Print and shaded views of the part. All mm, measured from the part's lowest x, y and z. A direction names the side the tool comes from. Give positions to 0.01 mm unless a question says otherwise; leave off trailing zeros. Loops run counter-clockwise (first coordinate to the right, second up) from the corner with the lowest first, then second, coordinate; pieces in that order, holes last. Notation, with made-up numbers: (-4.5, 4) -> (43.5, 4) arc R8 ccw to (43.5, 17) -> close; hole circle Ø5 at (7.5, 14). An arc over 180 degrees is marked (long way). Answer as a JSON object with one key per item and string values. Group by question number.
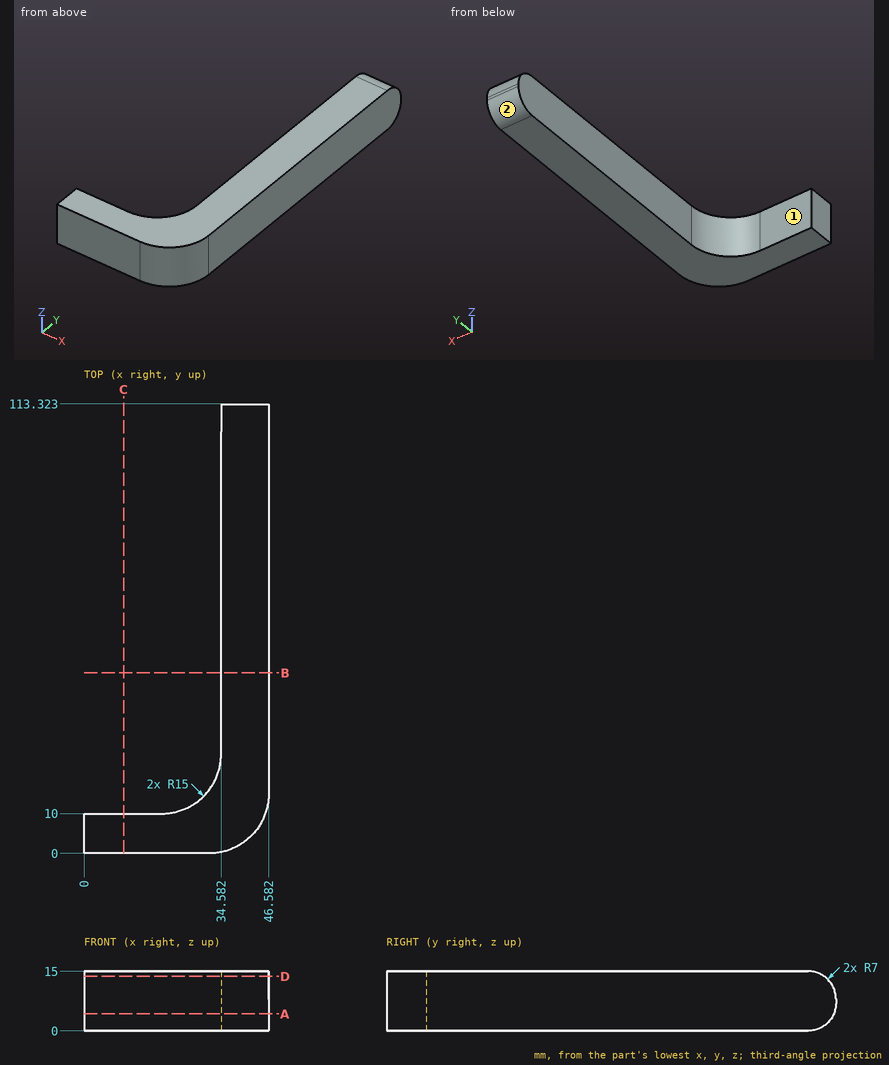
(1) Saw through at C-C on x = 10. List the corners of the cut face in (y, z).
(2) Probe line 1 along X through (y, z) = (26, 10.75); line 2 along Y through (x, z) = (8.5, 12); line 3 along Y through (x, z) = (21, 13.5). List the from-to ranges inside material, lowest first. Write a range as [from, to].
(3) Saw through at A-A on z = 4.25. List the corners of the cut face in (x, y), plus the area to 3 significant figures.
(4) Saw through at B-B on y = 45.5. List the corners of the cut face in (x, z).
(5) 3-axis set-ups, long thin cutter, end or side, ignore diameter. For the marked faces 1 and 2: which of +Z, -Z, +X, -X, +Y, -Y reach the whole face in a straight line?
(6) Pin check, flat tips, straight feed: pin 1 (8 mm diameter, centred on x = 9.5, z = 13, fed in from +Y); pin 2 (6 mm diameter, centred on x = 36, z = 12, fed in from -Y). Stop position of each tip, or through.
(7) Saw through at D-D on z = 13.75. List the corners of the cut face in (x, y) (1 decimal).
Calculated:
{
 "1": {"outline": "(0, 0) -> (10, 0) -> (10, 15) -> (0, 15) -> close"},
 "2": {"line 1": "x = [34.58, 46.58]", "line 2": "y = [0, 10]", "line 3": "y = [0, 10.07]"},
 "3": {"outline": "(0, 0) -> (31.58, 0) arc R15 ccw to (46.58, 15) -> (46.58, 112.76) -> (34.58, 112.76) -> (34.58, 25) arc R15 cw to (19.58, 10) -> (0, 10) -> close", "area": "1,700 mm^2"},
 "4": {"outline": "(34.58, 0) -> (46.58, 0) -> (46.58, 15) -> (34.58, 15) -> close"},
 "5": {"face 1": "+Z, -Z, -X, +Y", "face 2": "-Z, +X, -X, +Y"},
 "6": {"pin 1": "stops at y = 10", "pin 2": "stops at y = 0.07"},
 "7": {"outline": "(0, 0) -> (31.6, 0) arc R15 ccw to (46.6, 15) -> (46.6, 110.3) -> (34.6, 110.3) -> (34.6, 25) arc R15 cw to (19.6, 10) -> (0, 10) -> close"}
}
